The model under review builds one solid part; all positions refer to its coordinate system, in mm. A direction names the side the tool comes from. Give positions to 0.01 mm unless a question says otherwise; leave off trailing zeros. Write each loop counter-clockwise with the first axis right and the second up, starting at its lowest first coordinate (ties: lowest second). Pieces come first, ordered by that corner, then holes. Notation, with made-up numbers: (-28.5, 75) -> (10.5, 75) arc R32 ccw to (10.5, 111) -> close; hole circle Ø5 at (-40, 85.5). An arc over 180 degrees is marked (long way). Use CSV: the item, a comma, the result in double quotes.
```python
from build123d import *

# Parameters (mm, degrees)
SKETCH1_R                      = 40
SKETCH1_R_2                    = 4.3
SKETCH1_R_3                    = 30.1
SKETCH1_R_4                    = 4
BOSS_EXTRUDE1_DEPTH            = 39.7
CUT_EXTRUDE2_OUTLINE_R         = 4
CUT_EXTRUDE2_DEPTH             = 11
SKETCH2_R                      = 40
BOSS_EXTRUDE2_DEPTH            = 1
SKETCH3_R                      = 19.9
BOSS_EXTRUDE3_DEPTH            = 40.7
CUT_EXTRUDE3_DEPTH             = 3.2
CUT_EXTRUDE4_DEPTH             = 10
SKETCH6_R                      = 17.9
CUT_EXTRUDE5_DEPTH             = 63.898728127
SKETCH7_R                      = 0.8
CUT_EXTRUDE6_DEPTH             = 68.869359802
BOSS_EXTRUDE4_START            = -5
SKETCH8_R                      = 50
SKETCH8_R_2                    = 40
BOSS_EXTRUDE4_DEPTH            = 5
CBORE_FOR_M3_SHCS1_D           = 3.4
CBORE_FOR_M3_SHCS1_DEPTH       = 5
CBORE_FOR_M3_SHCS1_CBORE_D     = 6.5
CBORE_FOR_M3_SHCS1_CBORE_DEPTH = 3
CBORE_FOR_M3_SHCS1_TIP         = 1.021463052


# Read off the part's stored shape, not the designer's step: Cut-Extrude2
with BuildPart() as part:
    # Sketch1 → Boss-Extrude1 (new body)
    # profile 1 of 7: a face of its own
    with BuildSketch(Plane.XZ.offset(96.9)):
        with Locations(Location((0, 0, 0), (0, 0, 180))):
            Circle(SKETCH1_R)
        with Locations((0.154088268, -34.99966081)):
            Circle(SKETCH1_R_2, mode=Mode.SUBTRACT)
        with Locations((-34.494694465, 5.925879997)):
            Circle(SKETCH1_R_2, mode=Mode.SUBTRACT)
        with Locations((30.233551251, 17.63327476)):
            Circle(SKETCH1_R_2, mode=Mode.SUBTRACT)
        with Locations(Location((0, 0, 0), (0, 0, 180))):
            Circle(SKETCH1_R_3, mode=Mode.SUBTRACT)
    # profile 2 of 7: a face of its own
    with BuildSketch(Plane.XZ.offset(96.9)):
        with Locations((30.233551251, 17.63327476)):
            Circle(SKETCH1_R_2)
        with Locations((30.233551251, 17.63327476)):
            Circle(SKETCH1_R_4, mode=Mode.SUBTRACT)
    # profile 3 of 7: a face of its own
    with BuildSketch(Plane.XZ.offset(96.9)):
        with Locations((30.233551251, 17.63327476)):
            Circle(SKETCH1_R_4)
    # profile 4 of 7: a face of its own
    with BuildSketch(Plane.XZ.offset(96.9)):
        with Locations((-34.494694465, 5.925879997)):
            Circle(SKETCH1_R_2)
        with Locations((-34.494694465, 5.925879997)):
            Circle(SKETCH1_R_4, mode=Mode.SUBTRACT)
    # profile 5 of 7: a face of its own
    with BuildSketch(Plane.XZ.offset(96.9)):
        with Locations((-34.494694465, 5.925879997)):
            Circle(SKETCH1_R_4)
    # profile 6 of 7: a face of its own
    with BuildSketch(Plane.XZ.offset(96.9)):
        with Locations((0.154088268, -34.99966081)):
            Circle(SKETCH1_R_2)
        with Locations((0.154088268, -34.99966081)):
            Circle(SKETCH1_R_4, mode=Mode.SUBTRACT)
    # profile 7 of 7: a face of its own
    with BuildSketch(Plane.XZ.offset(96.9)):
        with Locations((0.154088268, -34.99966081)):
            Circle(SKETCH1_R_4)
    extrude(amount=BOSS_EXTRUDE1_DEPTH)

    # Cut-Extrude2 outline → Cut-Extrude2 (cut)
    with BuildSketch(Plane.XZ.offset(96.9)):
        with Locations((30.233551251, 17.63327476)):
            Circle(CUT_EXTRUDE2_OUTLINE_R)
        with Locations((0.154088268, -34.99966081)):
            Circle(CUT_EXTRUDE2_OUTLINE_R)
        with Locations((-34.494694465, 5.925879997)):
            Circle(CUT_EXTRUDE2_OUTLINE_R)
    extrude(amount=CUT_EXTRUDE2_DEPTH, mode=Mode.SUBTRACT)

    # Sketch2 → Boss-Extrude2 (add)
    with BuildSketch(Plane.XZ.offset(136.6)):
        Circle(SKETCH2_R)
    extrude(amount=BOSS_EXTRUDE2_DEPTH)

    # Sketch3 → Boss-Extrude3 (add)
    with BuildSketch(Plane.XZ.offset(137.6)):
        Circle(SKETCH3_R)
    extrude(amount=-BOSS_EXTRUDE3_DEPTH)

    # Sketch4 → Cut-Extrude3 (cut)
    with BuildSketch(Plane(origin=(0, -96.9, 0), x_dir=(1, 0, 0), z_dir=(0, 1, 0))):
        with BuildLine():
            Line((-5.48759728, 15.460346086), (-6.425775043, 15.806499932))
            Line((-6.425775043, 15.806499932), (-15.152313504, -7.844961471))
            Line((-15.152313504, -7.844961471), (-14.214135741, -8.191115317))
            ThreePointArc((-14.214135741, -8.191115317), (-12.734075949, -11.401944339), (-9.523246927, -9.921884547))
            Line((-9.523246927, -9.921884547), (-8.585069164, -10.268038394))
            Line((-8.585069164, -10.268038394), (0.141469298, 13.383423009))
            Line((0.141469298, 13.383423009), (-0.796708465, 13.729576855))
            ThreePointArc((-0.796708465, 13.729576855), (-2.276768257, 16.940405878), (-5.48759728, 15.460346086))
        make_face()
        with BuildLine():
            Line((-6.708713638, -10.960346086), (-7.646891401, -10.61419224))
            Line((-7.646891401, -10.61419224), (1.079647061, 13.037269163))
            Line((1.079647061, 13.037269163), (2.017824824, 12.691115317))
            ThreePointArc((2.017824824, 12.691115317), (5.228653846, 14.171175109), (6.708713638, 10.960346086))
            Line((6.708713638, 10.960346086), (7.646891401, 10.61419224))
            Line((7.646891401, 10.61419224), (-1.079647061, -13.037269163))
            Line((-1.079647061, -13.037269163), (-2.017824824, -12.691115317))
            ThreePointArc((-2.017824824, -12.691115317), (-5.228653846, -14.171175109), (-6.708713638, -10.960346086))
        make_face()
        with BuildLine():
            Line((6.425775043, -15.806499932), (5.48759728, -15.460346086))
            ThreePointArc((5.48759728, -15.460346086), (2.276768257, -16.940405878), (0.796708465, -13.729576855))
            Line((0.796708465, -13.729576855), (-0.141469298, -13.383423009))
            Line((-0.141469298, -13.383423009), (8.585069164, 10.268038394))
            Line((8.585069164, 10.268038394), (9.523246927, 9.921884547))
            ThreePointArc((9.523246927, 9.921884547), (12.734075949, 11.401944339), (14.214135741, 8.191115317))
            Line((14.214135741, 8.191115317), (15.152313504, 7.844961471))
            Line((15.152313504, 7.844961471), (6.425775043, -15.806499932))
        make_face()
    extrude(amount=-CUT_EXTRUDE3_DEPTH, mode=Mode.SUBTRACT)

    # Sketch5 → Cut-Extrude4 (cut)
    with BuildSketch(Plane(origin=(0, -100.1, 0), x_dir=(1, 0, 0), z_dir=(0, 1, 0))):
        Polygon((14.446159658, 5.931078834), (7.878915318, 8.354155757), (0.564684548, -11.469540373), (7.131928889, -13.892617296), align=None)
        Polygon((-7.131928889, 13.892617296), (-14.446159658, -5.931078834), (-7.878915318, -8.354155757), (-0.564684548, 11.469540373), align=None)
        Polygon((-0.373493214, -11.123386527), (6.940737555, 8.700309603), (0.373493214, 11.123386527), (-6.940737555, -8.700309603), align=None)
    extrude(amount=-CUT_EXTRUDE4_DEPTH, mode=Mode.SUBTRACT)

    # Sketch6 → Cut-Extrude5 (cut, through all)
    with BuildSketch(Plane(origin=(0, -110.1, 0), x_dir=(1, 0, 0), z_dir=(0, 1, 0))):
        with Locations(Location((0, 0, 0), (0, 0, 270))):
            Circle(SKETCH6_R)
    extrude(amount=-CUT_EXTRUDE5_DEPTH, mode=Mode.SUBTRACT)

    # Sketch7 → Cut-Extrude6 (cut, through all)
    with BuildSketch(Plane(origin=(0, -100.1, 0), x_dir=(1, 0, 0), z_dir=(0, 1, 0))):
        with Locations(Location((3.142152872, -14.594961471, 0), (0, 0, 180))):
            Circle(SKETCH7_R)
        with Locations(Location((-4.363269231, -11.825730701, 0), (0, 0, 180))):
            Circle(SKETCH7_R)
        with Locations(Location((-11.868691334, -9.056499932, 0), (0, 0, 180))):
            Circle(SKETCH7_R)
        with Locations(Location((-3.142152872, 14.594961471, 0), (0, 0, 180))):
            Circle(SKETCH7_R)
        with Locations(Location((4.363269231, 11.825730701, 0), (0, 0, 180))):
            Circle(SKETCH7_R)
        with Locations(Location((11.868691334, 9.056499932, 0), (0, 0, 180))):
            Circle(SKETCH7_R)
    extrude(amount=-CUT_EXTRUDE6_DEPTH, mode=Mode.SUBTRACT)

    # Sketch8 → Boss-Extrude4 (add)
    with BuildSketch(Plane.XZ.offset(137.6).offset(BOSS_EXTRUDE4_START)):
        Circle(SKETCH8_R)
        Circle(SKETCH8_R_2, mode=Mode.SUBTRACT)
    extrude(amount=BOSS_EXTRUDE4_DEPTH)

    # CBORE for M3 SHCS1
    with Locations(Plane(origin=(0, -132.6, 0), x_dir=(1, 0, 0), z_dir=(0, 1, 0))):
        with Locations((-40.867181552, -18.838085677), (-18.838085677, 40.867181552), (40.867181552, 18.838085677), (18.838085677, -40.867181552)):
            CounterBoreHole(CBORE_FOR_M3_SHCS1_D / 2, CBORE_FOR_M3_SHCS1_CBORE_D / 2, CBORE_FOR_M3_SHCS1_CBORE_DEPTH, depth=CBORE_FOR_M3_SHCS1_DEPTH)
            with Locations((0, 0, -(CBORE_FOR_M3_SHCS1_DEPTH + CBORE_FOR_M3_SHCS1_TIP / 2))):  # 118° drill point
                Cone(0, CBORE_FOR_M3_SHCS1_D / 2, CBORE_FOR_M3_SHCS1_TIP, mode=Mode.SUBTRACT)


solid = part.part
```
Q1. The part is to be moulded in two halves that separate along X. For faces 1 (the flat face through (4, -96.9, 0)), 2 (the cylindrical face through (47.69, -135.06, 15.02)), 3 (the cylindrical face through (-38.49, -102.32, 6.1)), say which applies: pulls with the +X half, pulls with the -X half, needs draft (parallel to the pull), parting line crosses it, or undercut.
Derived:
face 1,"needs draft"
face 2,"parting line crosses it"
face 3,"undercut"
Q2. Insertion check: pin 1 (6 mm diameter, centred on x = -17.5, y = -109.5, fed in from -Z); pin 2 (1.5 mm diameter, centred on y = -133, z = 35.5, fed in from -X); pin 3 (1 mm diameter, centred on x = 11.87, z = -9.06, fed in from +Y); pin 4 (10 mm diameter, centred on y = -118.5, z = 3.5, fed in from +X). Each pin has a flat end and moves straight along its axis. Give the tip position at first contact, or say it passes through.
Derived:
pin 1,"stops at z = -37.28"
pin 2,"stops at x = -35.95"
pin 3,"passes through"
pin 4,"stops at x = 40"
Q3. Consider section B-B (y = -117.5). Write out the cut boundary in (x, z).
Derived:
outline,"circle Ø80 at (0, 0); circle Ø39.8 at (0, 0); hole circle Ø60.2 at (0, 0); hole circle Ø35.8 at (0, 0)"
Q4. To check wall thickness, follow probe 1 along Z at (x, y) = (0.5, -132); probe 2 along X at (y, z) = (-110.5, -8.5); probe 3 along X at (y, z) = (-118, 2.5). State the ranges of each line that lie inside material, in increasing order.
Derived:
probe 1,"z = -40 to -30.1, -19.89 to -17.89, 17.89 to 19.89, 30.1 to 40"
probe 2,"x = -39.09 to -28.87, -17.99 to -15.75, 15.75 to 17.99, 28.87 to 39.09"
probe 3,"x = -39.92 to -30, -19.74 to -17.72, 17.72 to 19.74, 30 to 39.92"
Q5. Machinability: for faces 4 (the flat face through (11.209, -105.03, -7.126)), 5 (the flat face through (-17, -135.6, -39)), 6 (the cylindrical face through (17.748, -123.658, -2.33)), which of the approach directions +Z, -Z, +X, -X, +Y, -Y give a long, thin tool a straight path to every point of the face, cutting with its end or side? Answer none if there is none.
Derived:
face 4,"+Y, -Y"
face 5,"+Y"
face 6,"-Y"
Q6. Consider section A-A (y = -101.5). State how many separate pieces and enclosed holes the cut face has, then the cut area to 3 significant figures.
Derived:
separate pieces,"2"
enclosed holes,"13"
area,"2,820 mm2"
Q7. Consider section C-C (x = -33). Write out the cut boundary in (y, z), then the cut area to 3 significant figures.
Derived:
outline,"(-137.6, -37.56) -> (-132.6, -37.56) -> (-132.6, -22.61) -> (-96.9, -22.61) -> (-96.9, 2.22) -> (-107.9, 2.22) -> (-107.9, 9.64) -> (-96.9, 9.64) -> (-96.9, 22.61) -> (-132.6, 22.61) -> (-132.6, 37.56) -> (-137.6, 37.56) -> close"
area,"1,910 mm2"
